```python
from build123d import *

# Parameters (mm, degrees)
SKETCH1_W                = 46
SKETCH1_H                = 46
SKETCH1_R                = 3
SKETCH1_R_2              = 0.75
BOSS_EXTRUDE1_DEPTH      = 3
SKETCH2_W                = 46
SKETCH2_H                = 3
BOSS_EXTRUDE2_DEPTH      = 60
BOSS_EXTRUDE2_DEPTH_BACK = 3
SKETCH3_R                = 2
CUT_EXTRUDE1_DEPTH       = 10
SKETCH4_W                = 3
SKETCH4_H                = 60
SKETCH4_H_2              = 30
BOSS_EXTRUDE3_DEPTH      = 46
CUT_EXTRUDE2_DEPTH       = 46
CUT_EXTRUDE2_DEPTH_BACK  = 46
CUT_EXTRUDE3_DEPTH       = 15
SKETCH7_W                = 4.5
SKETCH7_H                = 3
CUT_EXTRUDE4_DEPTH       = 10


with BuildPart() as part:
    # Sketch1 → Boss-Extrude1 (new body)
    with BuildSketch(Plane.XY):
        with Locations((23, 23)):
            Rectangle(SKETCH1_W, SKETCH1_H)
        with Locations((23, 23)):
            Circle(SKETCH1_R, mode=Mode.SUBTRACT)
        with Locations((30, 23)):
            Circle(SKETCH1_R_2, mode=Mode.SUBTRACT)
        with Locations((23, 30)):
            Circle(SKETCH1_R_2, mode=Mode.SUBTRACT)
        with Locations((16, 23)):
            Circle(SKETCH1_R_2, mode=Mode.SUBTRACT)
        with Locations((23, 16)):
            Circle(SKETCH1_R_2, mode=Mode.SUBTRACT)
    extrude(amount=BOSS_EXTRUDE1_DEPTH)

    # Sketch2 → Boss-Extrude2 (add, two sides)
    with BuildSketch(Plane.XY.offset(3)) as boss_extrude2_sk:
        with Locations((23, 47.5)):
            Rectangle(SKETCH2_W, SKETCH2_H)
    extrude(amount=BOSS_EXTRUDE2_DEPTH)
    extrude(boss_extrude2_sk.sketch, amount=-BOSS_EXTRUDE2_DEPTH_BACK)

    # Sketch3 → Cut-Extrude1 (cut)
    with BuildSketch(Plane(origin=(0, 46, 0), x_dir=(-1, 0, 0), z_dir=(0, -1, 0))):
        with Locations((-18, -8.581054425)):
            Circle(SKETCH3_R)
        with Locations((-18, -57.381054425)):
            Circle(SKETCH3_R)
        with Locations((-28, -57.381054425)):
            Circle(SKETCH3_R)
        with Locations((-28, -8.581054425)):
            Circle(SKETCH3_R)
        Polygon((-22.5, -12.981054425), (-22.5, -8.581054425), (-23.5, -8.581054425), (-23.5, -12.981054425), (-33, -12.981054425), (-33, -52.981054425), (-23.5, -52.981054425), (-23.5, -57.381054425), (-22.5, -57.381054425), (-22.5, -52.981054425), (-13, -52.981054425), (-13, -12.981054425), align=None)
    extrude(amount=-CUT_EXTRUDE1_DEPTH, mode=Mode.SUBTRACT)

    # Sketch4 → Boss-Extrude3 (add)
    with BuildSketch(Plane(origin=(0, 46, 0), x_dir=(-1, 0, 0), z_dir=(0, -1, 0))):
        with Locations((-44.5, -33)):
            Rectangle(SKETCH4_W, SKETCH4_H)
        with Locations((-1.5, -18)):
            Rectangle(SKETCH4_W, SKETCH4_H_2)
    extrude(amount=BOSS_EXTRUDE3_DEPTH)

    # Sketch5 → Cut-Extrude2 (cut, two sides)
    with BuildSketch(Plane.ZY.offset(-43)) as cut_extrude2_sk:
        Polygon((63, 46), (3, 0), (63, 0), align=None)
    extrude(amount=CUT_EXTRUDE2_DEPTH, mode=Mode.SUBTRACT)
    extrude(cut_extrude2_sk.sketch, amount=-CUT_EXTRUDE2_DEPTH_BACK, mode=Mode.SUBTRACT)

    # Sketch6 → Cut-Extrude3 (cut)
    with BuildSketch(Plane.ZY):
        Polygon((3, 0), (33, 46), (33, 23), align=None)
    extrude(amount=-CUT_EXTRUDE3_DEPTH, mode=Mode.SUBTRACT)

    # Sketch7 → Cut-Extrude4 (cut)
    with BuildSketch(Plane.XY.offset(3)):
        with Locations((36.25, 38.5)):
            Rectangle(SKETCH7_W, SKETCH7_H)
        with Locations((31.75, 38.5)):
            Rectangle(SKETCH7_W, SKETCH7_H)
    extrude(amount=-CUT_EXTRUDE4_DEPTH, mode=Mode.SUBTRACT)


solid = part.part
```
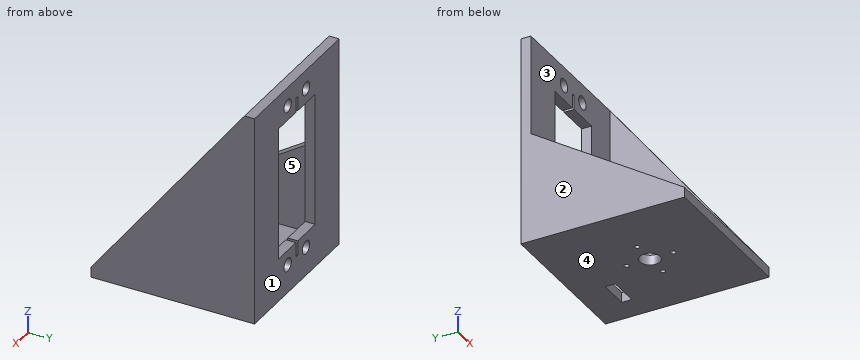
For this review, take the finished solid that the model builds, in its own axes (mm). Face numbers are marked on the shaded views. A direction names the side the tool comes from. Round coordinates to 2 decimals unless told otherwise and drop trailing zeros. Write each loop counter-clockwise with the first axis right and the second up, starting at its lowest first coordinate (ties: lowest second). Pieces come first, ordered by that corner, then holes. Notation, with made-up numbers: (46, 64.5) -> (95, 64.5) arc R17 ccw to (95, 68.5) -> close; hole circle Ø10 at (25.5, -1). An arc over 180 degrees is marked (long way). One line per question, with ' | ' between items. Start each with the question number.
1) Mouldability with a two-part tool opening along X and no side actions: class the marked faces 1, 2 and 3 as +X half, -X half, draft (parallel to the pull), parting line (faces both ways), or undercut.
2) Machinability: for the marked faces 4 and 5, which of the approach directions +Z, -Z, +X, -X, +Y, -Y give a long, thin tool a straight path to every point of the face, cutting with its end or side? Answer none if there is none.
3) Add section A-A (x = 18). Write out the cut boundary in (y, z), and give its area (3 significant figures).
4) For pin 1 Ø8 at (x, z) = (7.5, 19) entering from -Y; pin 2 Ø2 at (y, z) = (41, 36.5) entering from -X; pin 3 Ø12 at (x, y) = (16.5, 19.5) entering from +Z, all flat-tipped, find the tip position at first contact; note any pin that passes through.
5) Add section B-B (z = 18.5). Write out the cut boundary in (x, y), and give its area (3 significant figures).
6) Wall thickness on line 1 along Y through (x, z) = (23, 1); line 2 along X through (y, z) = (25.5, 10); line 3 along Z through (x, y) = (31, 28.5): over which ranges is each line inside the solid? List them lowest first.
7) Add section D-D (y = 35.5). Write out the cut boundary in (x, z).
8) Add section C-C (y = 16). Write out the cut boundary in (x, z), and give its area (3 significant figures).
Reported:
1) face 1: draft | face 2: -X half | face 3: undercut
2) face 4: -Z, +X, -X, +Y, -Y | face 5: +Z, -Y
3) outline: (0, 0) -> (49, 0) -> (49, 6.58) -> (46, 6.58) -> (46, 3) -> (0, 3) -> close; (46, 10.58) -> (49, 10.58) -> (49, 12.98) -> (46, 12.98) -> close; (46, 52.98) -> (49, 52.98) -> (49, 55.38) -> (46, 55.38) -> close; (46, 59.38) -> (49, 59.38) -> (49, 63) -> (46, 63) -> close | area: 183 mm²
4) pin 1: stops at y = 46 | pin 2: stops at x = 43 | pin 3: stops at z = 3
5) outline: (0, 23.77) -> (3, 23.77) -> (3, 46) -> (13, 46) -> (13, 49) -> (0, 49) -> close; (33, 46) -> (43, 46) -> (43, 11.88) -> (46, 11.88) -> (46, 49) -> (33, 49) -> close | area: 247 mm²
6) line 1: y = 0 to 15.25, 16.75 to 20, 26 to 29.25, 30.75 to 49 | line 2: x = 0 to 3, 43 to 46 | line 3: z = 0 to 3
7) outline: (0, 0) -> (46, 0) -> (46, 49.3) -> (43, 49.3) -> (43, 3) -> (3, 3) -> (3, 26.15) -> (0, 26.15) -> close
8) outline: (0, 0) -> (22.25, 0) -> (22.25, 3) -> (3, 3) -> (3, 13.43) -> (0, 13.43) -> close; (23.75, 0) -> (46, 0) -> (46, 23.87) -> (43, 23.87) -> (43, 3) -> (23.75, 3) -> close | area: 227 mm²
